Work out the finished part from the listing and answer in its coordinate system (mm). Face numbers are marked on the shaded views. A direction names the side the tool comes from. Coordinates: 2 decimals unless noted, no trailing zeros. Order: outer loops, then holes, each group sorted by start corner. A loop starts at its lowest first (then second) coordinate and runs counter-clockwise, first axis right, second up.
1. The part is cut by section A-A, the plane y = 20.5. Give the vertices of the cut face in (x, z).
2. Find the intervals of material crossed by probe 1 along Y at (x, z) = (82, 25.5); probe 2 along Z at (x, y) = (87, -8); probe 3 along Z at (x, y) = (-149.5, -4), in increasing order.
3. Determine the mould class of the marked faces 1, 2 and 3 for opening direction Y: +Y half, -Y half, draft (parallel to the pull), parting line (faces both ways), or undercut.
4. The part is cut by section C-C, the plane x = 125.5. Give the vertices of the cut face in (y, z).
5. A tool of negligible diameter and unlimited length cuts with its end or side. For the marked faces 4 and 5, from which of +Z, -Z, +X, -X, +Y, -Y can it reach the whole face along a straight path? Write none if from no direction.
6. The part is cut by section B-B, the plane z = 27.5. Give the vertices of the cut face in (x, y), then the cut area to 3 significant figures.
```python
from build123d import *

# Parameters (mm, degrees)
F1_DEPTH = 209.55


with BuildPart() as f1:
    # F0 (on Right) → F1 (new body, symmetric)
    with BuildSketch(Plane.YZ):
        Polygon((69.85, 50.8), (-69.85, 50.8), (-69.85, 0), (-0.127, 0), (-0.127, 45.7835), (-4.7625, 45.7835), (-4.7625, 4.7625), (-65.0875, 4.7625), (-65.0875, 46.0375), (65.0875, 46.0375), (65.0875, 4.7625), (4.7625, 4.7625), (4.7625, 45.7835), (0.127, 45.7835), (0.127, 0), (69.85, 0), align=None)
    extrude(amount=F1_DEPTH, both=True)


solid = f1.part
```
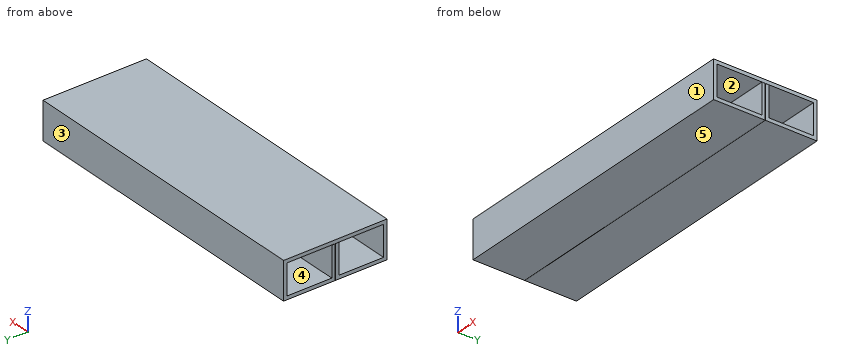
Geometry says:
1. outline: (-209.55, 0) - (209.55, 0) - (209.55, 4.76) - (-209.55, 4.76) - close; (-209.55, 46.04) - (209.55, 46.04) - (209.55, 50.8) - (-209.55, 50.8) - close
2. probe 1: y = -69.85 to -65.09, -4.76 to -0.13, 0.13 to 4.76, 65.09 to 69.85
2. probe 2: z = 0 to 4.76, 46.04 to 50.8
2. probe 3: z = 0 to 45.78, 46.04 to 50.8
3. face 1: -Y half
3. face 2: undercut
3. face 3: +Y half
4. outline: (-69.85, 0) - (-0.13, 0) - (-0.13, 45.78) - (-4.76, 45.78) - (-4.76, 4.76) - (-65.09, 4.76) - (-65.09, 46.04) - (65.09, 46.04) - (65.09, 4.76) - (4.76, 4.76) - (4.76, 45.78) - (0.13, 45.78) - (0.13, 0) - (69.85, 0) - (69.85, 50.8) - (-69.85, 50.8) - close
5. face 4: +X, -X
5. face 5: -Z, +X, -X, +Y, -Y
6. outline: (-209.55, -69.85) - (209.55, -69.85) - (209.55, -65.09) - (-209.55, -65.09) - close; (-209.55, -4.76) - (209.55, -4.76) - (209.55, -0.13) - (-209.55, -0.13) - close; (-209.55, 0.13) - (209.55, 0.13) - (209.55, 4.76) - (-209.55, 4.76) - close; (-209.55, 65.09) - (209.55, 65.09) - (209.55, 69.85) - (-209.55, 69.85) - close
6. area: 7,880 mm2
